The listing builds one solid part. Answer for the finished solid, in the listing's coordinates (mm). Face numbers are marked on the shaded views. A direction names the side the tool comes from. Round coordinates to 2 decimals unless told otherwise and drop trailing zeros. Loops run counter-clockwise (first coordinate to the right, second up) from the corner with the lowest first, then second, coordinate; pieces in that order, holes last. Notation, with made-up numbers: (43, -9) -> (66, -9) arc R33 ccw to (66, 21) -> close; hole circle Ø8 at (0, -34). An arc over 180 degrees is marked (long way). Write each question's results on one line, items separated by ' | '. Start each with the question number.
(1) The part is cut by section B-B (z = -7.5). Determine the outline of the cut face in (x, y).
(2) Flat-ended cylindrical pins translate along their axes: pin 1 (10 mm diameter, centred on y = -19.5, z = 15.5, fed in from +X); pin 2 (3.5 mm diameter, centred on y = -13.5, z = -31.5, fed in from -X); pin 3 (7.5 mm diameter, centred on y = -14, z = -39.5, fed in from +X). Find the tip coordinate at first contact, or state that the pin passes through.
(3) Straight lines are drawn through the part: probe 1 along Y at (x, z) = (31.75, -35.1); probe 2 along Z at (x, y) = (-36, -22.75); probe 3 along X at (y, z) = (-2.5, 30.5). For each, find the intervals that lie inside material, in ascending order.
(4) For the marked faces 1, 2, 3 and 4, determine the directions among +Z, -Z, +X, -X, +Y, -Y from which every point of the face is accessible in a straight line to the end or side of a thin tool.
(5) Determine the mould class of the marked faces 5, 6, 7 and 8 for opening direction Z: released by +Z, released by -Z, zero draft, split by the parting line, or undercut.
(6) The part is cut by section A-A (x = -33.5). Determine the outline of the cut face in (y, z).
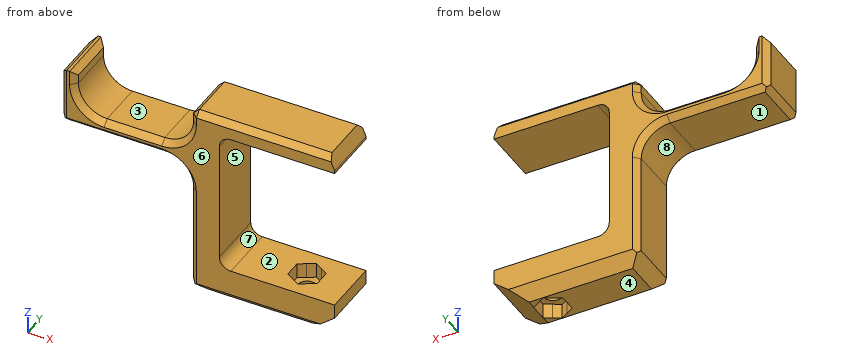
```python
from build123d import *

# Parameters (mm, degrees)
F0_W       = 50.8
F0_H       = 6.35
F0_H_2     = 7.62
F0_H_3     = 16.51
F1_DEPTH   = 25.4
F2_R       = 12.7
F3_SIZE    = 2.54
F4_R       = 12.7
F5_SIZE    = 2.54
F6_R       = 5.08
F8_C1_SIZE = 5.08
F8_C2_SIZE = 5.08
F8_C3_SIZE = 5.08
F9_SIZE2   = 12.7
F9_SIZE    = 10.16
F10_SIZE2  = 6.35
F10_SIZE   = 2.54
F11_DEPTH  = 6.604
F12_START  = -9.906
F12_DEPTH  = 6.605
F13_D      = 8.128
F13_DEPTH  = 16.511


with BuildPart() as f1:
    # F0 (on Front) → F1 (new body)
    with BuildSketch(Plane.XZ):
        Polygon((-63.5, 19.1297054841), (-63.5, 25.4797054841), (-63.5, 44.5297054841), (-69.85, 44.5297054841), (-69.85, 19.1297054841), align=None)
        with Locations((-38.1, 22.3047054841)):
            Rectangle(F0_W, F0_H)
        Polygon((0, 36.9097054841), (0, 44.5297054841), (-12.7, 44.5297054841), (-12.7, 25.4797054841), (-12.7, 19.1297054841), (-12.7, -43.1002945159), (0, -43.1002945159), (0, -26.5902945159), align=None)
        with Locations((25.4, 40.7197054841)):
            Rectangle(F0_W, F0_H_2)
        with Locations((25.4, -34.8452945159)):
            Rectangle(F0_W, F0_H_3)
    extrude(amount=F1_DEPTH)

    # F2
    f2_edges = [f1.edges().sort_by_distance(p)[0] for p in [
        (-12.7, -12.7, 25.479705),
        (-63.5, -12.7, 25.479705),
    ]]
    fillet(f2_edges, radius=F2_R)

    # F3
    f3_edges = [f1.edges().sort_by_distance(p)[0] for p in [
        (-63.5, -12.7, 44.529705),
        (-69.85, 0, 31.829705),
        (-69.85, -12.7, 44.529705),
        (-69.85, -25.4, 31.829705),
        (-59.780256, -25.4, 29.199449),
        (-38.1, 0, 25.479705),
        (-12.7, -12.7, 44.529705),
        (19.05, -25.4, 44.529705),
        (19.05, 0, 44.529705),
        (-69.85, -12.7, 19.129705),
    ]]
    chamfer(f3_edges, length=F3_SIZE)

    # F4
    f4_edges = [f1.edges().sort_by_distance(p)[0] for p in [
        (-12.7, -12.7, 19.129705),
    ]]
    fillet(f4_edges, radius=F4_R)

    # F5
    f5_edges = [f1.edges().sort_by_distance(p)[0] for p in [
        (-12.7, -25.4, -18.335295),
        (-12.7, 0, -18.335295),
    ]]
    chamfer(f5_edges, length=F5_SIZE)

    # F6
    f6_edges = [f1.edges().sort_by_distance(p)[0] for p in [
        (0, -12.7, 36.909705),
        (0, -12.7, -26.590295),
    ]]
    fillet(f6_edges, radius=F6_R)

    # F8: chamfer of 5.08 on 5 edges, made by hand

    # F8_c1
    f8_c1_edges = [f1.edges().sort_by_distance(p)[0] for p in [
        (20.32, 0, -43.1002945159),
    ]]
    chamfer(f8_c1_edges, length=F8_C1_SIZE)

    # F8_c2
    f8_c2_edges = [f1.edges().sort_by_distance(p)[0] for p in [
        (-12.7, -13.97, -43.1002945159),
    ]]
    chamfer(f8_c2_edges, length=F8_C2_SIZE)

    # F8_c3
    f8_c3_edges = [f1.edges().sort_by_distance(p)[0] for p in [
        (21.59, -25.4, -43.1002945159),
    ]]
    chamfer(f8_c3_edges, length=F8_C3_SIZE)

    # F9
    f9_edges = [f1.edges().sort_by_distance(p)[0] for p in [
        (50.8, -12.7, -43.100295),
    ]]
    f9_side = f1.faces().sort_by_distance((50.8, -12.7, -34.415021))[0]
    chamfer(f9_edges, length=F9_SIZE, length2=F9_SIZE2, reference=f9_side)

    # F10
    f10_edges = [f1.edges().sort_by_distance(p)[0] for p in [
        (50.8, -12.7, 44.529705),
    ]]
    f10_side = f1.faces().sort_by_distance((20.32, -12.7, 44.529705))[0]
    chamfer(f10_edges, length=F10_SIZE, length2=F10_SIZE2, reference=f10_side)

    # F7 (on face) → F11 (cut)
    with BuildSketch(Plane.XY.offset(-26.5902945159)):
        with BuildLine():
            Line((25.273, -16.4394976935), (28.5114998927, -18.3092464784))
            ThreePointArc((28.5114998927, -18.3092464784), (26.1407534287, -15.9384999464), (25.273, -12.7))
            Line((25.273, -12.7), (25.273, -16.4394976935))
        make_face()
        with BuildLine():
            ThreePointArc((25.273, -12.7), (26.1407534711, -9.4614999803), (28.5115000394, -7.0907534369))
            Line((28.5115000394, -7.0907534369), (25.273, -8.9605023065))
            Line((25.273, -8.9605023065), (25.273, -12.7))
        make_face()
        with BuildLine():
            ThreePointArc((28.5115000394, -7.0907534369), (31.7500001819, -6.223), (34.9885002756, -7.0907536188))
            Line((34.9885002756, -7.0907536188), (31.75, -5.2210046129))
            Line((31.75, -5.2210046129), (28.5115000394, -7.0907534369))
        make_face()
        with BuildLine():
            ThreePointArc((34.9885002756, -7.0907536188), (37.3592466199, -9.4615001378), (38.227, -12.7))
            Line((38.227, -12.7), (38.227, -8.9605023065))
            Line((38.227, -8.9605023065), (34.9885002756, -7.0907536188))
        make_face()
        with BuildLine():
            Line((38.227, -16.4394976935), (38.227, -12.7))
            ThreePointArc((38.227, -12.7), (37.3592466025, -15.9384998923), (34.9885002155, -18.3092464159))
            Line((34.9885002155, -18.3092464159), (38.227, -16.4394976935))
        make_face()
        with BuildLine():
            Line((31.75, -20.1789953871), (34.9885002155, -18.3092464159))
            ThreePointArc((34.9885002155, -18.3092464159), (31.7500000625, -19.177), (28.5114998927, -18.3092464784))
            Line((28.5114998927, -18.3092464784), (31.75, -20.1789953871))
        make_face()
        with BuildLine():
            ThreePointArc((34.9885002155, -18.3092464159), (37.3592466025, -15.9384998923), (38.227, -12.7))
            ThreePointArc((38.227, -12.7), (37.3592466199, -9.4615001378), (34.9885002756, -7.0907536188))
            ThreePointArc((34.9885002756, -7.0907536188), (31.7500001819, -6.223), (28.5115000394, -7.0907534369))
            ThreePointArc((28.5115000394, -7.0907534369), (26.1407534711, -9.4614999803), (25.273, -12.7))
            ThreePointArc((25.273, -12.7), (26.1407534287, -15.9384999464), (28.5114998927, -18.3092464784))
            ThreePointArc((28.5114998927, -18.3092464784), (31.7500000625, -19.177), (34.9885002155, -18.3092464159))
        make_face()
    extrude(amount=-F11_DEPTH, mode=Mode.SUBTRACT)

    # F7 (on face) → F12 (cut)
    with BuildSketch(Plane.XY.offset(-26.5902945159).offset(F12_START)):
        with BuildLine():
            ThreePointArc((34.9885002155, -18.3092464159), (37.3592466025, -15.9384998923), (38.227, -12.7))
            ThreePointArc((38.227, -12.7), (37.3592466199, -9.4615001378), (34.9885002756, -7.0907536188))
            ThreePointArc((34.9885002756, -7.0907536188), (31.7500001819, -6.223), (28.5115000394, -7.0907534369))
            ThreePointArc((28.5115000394, -7.0907534369), (26.1407534711, -9.4614999803), (25.273, -12.7))
            ThreePointArc((25.273, -12.7), (26.1407534287, -15.9384999464), (28.5114998927, -18.3092464784))
            ThreePointArc((28.5114998927, -18.3092464784), (31.7500000625, -19.177), (34.9885002155, -18.3092464159))
        make_face()
        with BuildLine():
            Line((38.227, -16.4394976935), (38.227, -12.7))
            ThreePointArc((38.227, -12.7), (37.3592466025, -15.9384998923), (34.9885002155, -18.3092464159))
            Line((34.9885002155, -18.3092464159), (38.227, -16.4394976935))
        make_face()
        with BuildLine():
            ThreePointArc((28.5115000394, -7.0907534369), (31.7500001819, -6.223), (34.9885002756, -7.0907536188))
            Line((34.9885002756, -7.0907536188), (31.75, -5.2210046129))
            Line((31.75, -5.2210046129), (28.5115000394, -7.0907534369))
        make_face()
        with BuildLine():
            ThreePointArc((34.9885002756, -7.0907536188), (37.3592466199, -9.4615001378), (38.227, -12.7))
            Line((38.227, -12.7), (38.227, -8.9605023065))
            Line((38.227, -8.9605023065), (34.9885002756, -7.0907536188))
        make_face()
        with BuildLine():
            ThreePointArc((25.273, -12.7), (26.1407534711, -9.4614999803), (28.5115000394, -7.0907534369))
            Line((28.5115000394, -7.0907534369), (25.273, -8.9605023065))
            Line((25.273, -8.9605023065), (25.273, -12.7))
        make_face()
        with BuildLine():
            Line((25.273, -16.4394976935), (28.5114998927, -18.3092464784))
            ThreePointArc((28.5114998927, -18.3092464784), (26.1407534287, -15.9384999464), (25.273, -12.7))
            Line((25.273, -12.7), (25.273, -16.4394976935))
        make_face()
        with BuildLine():
            Line((31.75, -20.1789953871), (34.9885002155, -18.3092464159))
            ThreePointArc((34.9885002155, -18.3092464159), (31.7500000625, -19.177), (28.5114998927, -18.3092464784))
            Line((28.5114998927, -18.3092464784), (31.75, -20.1789953871))
        make_face()
    extrude(amount=-F12_DEPTH, mode=Mode.SUBTRACT)

    # F13 (through all, one way)
    with BuildSketch(Plane.XY.offset(-26.5902945159)):
        with Locations((31.75, -12.7)):
            Circle(F13_D / 2)
    extrude(amount=-F13_DEPTH, mode=Mode.SUBTRACT)


solid = f1.part
```
Checked values:
1) outline: (-12.7, -22.86) -> (-10.16, -25.4) -> (0, -25.4) -> (0, 0) -> (-10.16, 0) -> (-12.7, -2.54) -> close
2) pin 1: stops at x = 0 | pin 2: stops at x = -12.7 | pin 3: stops at x = 47.29
3) probe 1: y = -25.4 to -16.76, -8.64 to 0 | probe 2: z = 19.13 to 25.48 | probe 3: x = -69.81 to -60.97, -15.23 to 0
4) face 1: -Z, -X, +Y, -Y | face 2: +X, +Y, -Y | face 3: +Z, +Y, -Y | face 4: -Z, +X, -X, +Y, -Y
5) face 5: undercut | face 6: zero draft | face 7: undercut | face 8: released by -Z
6) outline: (-25.4, 21.67) -> (-22.86, 19.13) -> (-2.54, 19.13) -> (0, 21.67) -> (0, 22.94) -> (-2.54, 25.48) -> (-22.86, 25.48) -> (-25.4, 22.94) -> close
